Check sheet for the modelled part. Datum: model origin and axes. Units: mm. A direction names the side the tool comes from. Round coordinates to 2 decimals unless told otherwise and drop trailing zeros. Answer in a Markdown table with one row per item.
```python
from build123d import *

# Parameters (mm, degrees)
SKETCH2_OUTSIDE_W  = 36.282
SKETCH2_OUTSIDE_H  = 36.282
CUT_EXTRUDE1_DEPTH = 2.54
CUT_EXTRUDE2_DEPTH = 1.27


with BuildPart() as part:
    # Sketch1 → Revolve1 (revolve)
    with BuildSketch(Plane(origin=(0, 0, 0), x_dir=(0, 0, -1), z_dir=(1, 0, 0)), mode=Mode.PRIVATE) as revolve1_sk:
        Polygon((9.525, -0.925479408), (13.335, -0.925479408), (13.335, 3.773520592), (11.049, 4.154520592), (10.063815367, 4.154520592), (9.525, 3.615705224), (10.063815367, 3.076889857), (9.525, 2.53807449), (10.063815367, 1.999259122), (9.525, 1.460443755), (10.063815367, 0.921628388), (9.525, 0.382813021), (10.063815367, -0.156002347), (9.525, -0.694817714), align=None)
    revolve(revolve1_sk.sketch.rotate(Axis((0, 15.090367901, 0), (0, -1, 0)), 180), axis=Axis((0, 15.090367901, 0), (0, -1, 0)))

    # Sketch2 outside → Cut-Extrude1 (cut)
    with BuildSketch(Plane(origin=(0, 4.154520592, 0), x_dir=(-1, 0, 0), z_dir=(0, 1, 0))):
        Rectangle(SKETCH2_OUTSIDE_W, SKETCH2_OUTSIDE_H)
        Polygon((0, -13.335), (11.548448759, -6.6675), (11.548448759, 6.6675), (0, 13.335), (-11.548448759, 6.6675), (-11.548448759, -6.6675), align=None, mode=Mode.SUBTRACT)
    extrude(amount=-CUT_EXTRUDE1_DEPTH, mode=Mode.SUBTRACT)

    # Sketch3 → Cut-Extrude2 (cut)
    with BuildSketch(Plane.XZ.offset(0.925479408)):
        with BuildLine():
            Line((-4.7625, 8.248891971), (-6.6675, 11.548448759))
            ThreePointArc((-6.6675, 11.548448759), (-5.833267647, 11.991464196), (-4.969767422, 12.374313588))
            Line((-4.969767422, 12.374313588), (-3.620124564, 8.810239675))
            ThreePointArc((-3.620124564, 8.810239675), (-4.20069952, 8.548669402), (-4.7625, 8.248891971))
        make_face()
        with BuildLine():
            Line((2.465251405, 9.200443495), (3.451351966, 12.880620894))
            ThreePointArc((3.451351966, 12.880620894), (4.354502539, 12.603988759), (5.235804805, 12.264117296))
            Line((5.235804805, 12.264117296), (3.66996559, 8.789594847))
            ThreePointArc((3.66996559, 8.789594847), (3.074478988, 9.015165221), (2.465251405, 9.200443495))
        make_face()
        with BuildLine():
            Line((8.248891971, 4.7625), (11.548448759, 6.6675))
            ThreePointArc((11.548448759, 6.6675), (11.991464196, 5.833267647), (12.374313588, 4.969767422))
            Line((12.374313588, 4.969767422), (8.810239675, 3.620124564))
            ThreePointArc((8.810239675, 3.620124564), (8.548669402, 4.20069952), (8.248891971, 4.7625))
        make_face()
        with BuildLine():
            Line((9.200443495, -2.465251405), (12.880620894, -3.451351966))
            ThreePointArc((12.880620894, -3.451351966), (12.603988759, -4.354502539), (12.264117296, -5.235804805))
            Line((12.264117296, -5.235804805), (8.789594847, -3.66996559))
            ThreePointArc((8.789594847, -3.66996559), (9.015165221, -3.074478988), (9.200443495, -2.465251405))
        make_face()
        with BuildLine():
            Line((4.7625, -8.248891971), (6.6675, -11.548448759))
            ThreePointArc((6.6675, -11.548448759), (5.833267647, -11.991464196), (4.969767422, -12.374313588))
            Line((4.969767422, -12.374313588), (3.620124564, -8.810239675))
            ThreePointArc((3.620124564, -8.810239675), (4.20069952, -8.548669402), (4.7625, -8.248891971))
        make_face()
        with BuildLine():
            Line((-2.465251405, -9.200443495), (-3.451351966, -12.880620894))
            ThreePointArc((-3.451351966, -12.880620894), (-4.354502539, -12.603988759), (-5.235804805, -12.264117296))
            Line((-5.235804805, -12.264117296), (-3.66996559, -8.789594847))
            ThreePointArc((-3.66996559, -8.789594847), (-3.074478988, -9.015165221), (-2.465251405, -9.200443495))
        make_face()
        with BuildLine():
            Line((-8.248891971, -4.7625), (-11.548448759, -6.6675))
            ThreePointArc((-11.548448759, -6.6675), (-11.991464196, -5.833267647), (-12.374313588, -4.969767422))
            Line((-12.374313588, -4.969767422), (-8.810239675, -3.620124564))
            ThreePointArc((-8.810239675, -3.620124564), (-8.548669402, -4.20069952), (-8.248891971, -4.7625))
        make_face()
        with BuildLine():
            Line((-9.200443495, 2.465251405), (-12.880620894, 3.451351966))
            ThreePointArc((-12.880620894, 3.451351966), (-12.603988759, 4.354502539), (-12.264117296, 5.235804805))
            Line((-12.264117296, 5.235804805), (-8.789594847, 3.66996559))
            ThreePointArc((-8.789594847, 3.66996559), (-9.015165221, 3.074478988), (-9.200443495, 2.465251405))
        make_face()
    extrude(amount=-CUT_EXTRUDE2_DEPTH, mode=Mode.SUBTRACT)


solid = part.part
```
(1) Scan lines: probe 1 along X at (y, z) = (-0.2, -11); probe 2 along X at (y, z) = (3.9, -4.5); probe 3 along Z at (x, y) = (-10.5, -0.1). Record each from-to range of solid material in increasing order. Write a range as from..to.
Solutions:
| item | result |
|---|---|
| probe 1 | -7.54..-4.67, -2.95..4.45, 6.35..7.54 |
| probe 2 | -11.55..-8.72, 8.72..11.55 |
| probe 3 | -8.22..-6.06, -4.26..2.81, 4.44..8.22 |
(2) Depth check by flat-ended pin: pin 1 Ø1.5 at (y, z) = (0, 4.5) entering from +X; pin 2 Ø0.7 at (y, z) = (2.5, -3.5) entering from -X; pin 3 Ø2 at (x, z) = (12.5, -1) entering from +Y; pin 4 Ø1 at (x, z) = (7, -5.5) entering from -Y. Enter the tip coordinate at first touch or a pass-through.
Solutions:
| item | result |
|---|---|
| pin 1 | x = 12.8 |
| pin 2 | x = -11.55 |
| pin 3 | y = 4.07 |
| pin 4 | through |
(3) Draft check along Y on faces 6 (the conical face through (9.7, -0.5, 0.6)), 7 (the flat face through (-6.2, 1.615, -10.5)), 8 (the flat face through (-11, -0.925, -1)), 9 (the conical face through (0.6, -0.5, -9.7)). Enter one of: pulls with the +Y half, pulls with the -Y half, needs draft (parallel to the pull), parting line crosses it, or undercut.
Solutions:
| item | result |
|---|---|
| face 6 | undercut |
| face 7 | pulls with the +Y half |
| face 8 | pulls with the -Y half |
| face 9 | undercut |
(4) Tool access check on faces 1 (the flat face through (-6, 1.615, 11)), 2 (the flat face through (11.548, 3, 0)), 3 (the conical face through (-9.7, -0.5, -0.6)), 4 (the flat face through (-10.551, -0.299, 4.464)), 5 (the flat face through (4, 0.345, 11)). Record the directions out of +Z, -Z, +X, -X, +Y, -Y that give a thin tool (end or side, any length) a straight path to the whole face; none if there is none.
Solutions:
| item | result |
|---|---|
| face 1 | +Z, -X, +Y |
| face 2 | +Z, -Z, +X, +Y |
| face 3 | none |
| face 4 | -X, -Y |
| face 5 | -Y |
